Build history of the part. All positions in model axes, mm. A direction names the side the tool comes from. Round coordinates to 2 decimals unless told otherwise and drop trailing zeros. Write each loop counter-clockwise with the first axis right and the second up, starting at its lowest first coordinate (ties: lowest second). Pieces come first, ordered by that corner, then holes. Notation, with made-up numbers: (82, 73.25) - (99, 73.25) arc R36 ccw to (99, 109.25) - close; hole circle Ø3 at (-22.5, 61.5). An arc over 180 degrees is marked (long way). Answer as a JSON object with one key per item and string values. Group by question number.
Item 1: Slice it at A-A, the plane x = -105.5. List the corners of the cut face in (y, z), then the cut area to 3 significant figures.
Item 2: Flat gauge pins, fed straight in: pin 1 (2 mm diameter, centred on y = 37, z = 11.5, fed in from -X); pin 2 (1 mm diameter, centred on x = -4.5, z = 5.5, fed in from -Y); pin 3 (1.5 mm diameter, centred on x = 50.5, y = 78.5, fed in from +Z). Where does each tip first touch, or does it go through?
Item 3: Slice it at B-B, the plane z = 39. List the corners of the cut face in (x, y), then the cut area to 3 significant figures.
Item 4: Which spindle directions (+Z, -Z, +X, -X, +Y, -Y) get a long thin tool onto all of the face, cutting with end or side? Do faces 4 (the cylindrical face through (27.268, 57.226, -13.977)), 5 (the cylindrical face through (23.846, 14.79, 7.509)), 6 (the flat face through (-130, 100, 0)), 7 (the cylindrical face through (-114.79, 118.426, 16.896)). Say none if no direction does.
Item 5: Two-plate mould, pull along X, no slides. Class faces 1 (the flat face through (0, 109.6, 23.3)), 2 (the flat face through (0, 30, 0)), 3 (the flat face through (17, 0, -19)): +X half, -X half, draft (parallel to the pull), parting line (faces both ways), or undercut.
Item 6: Slice it at D-D, the plane z = 67.5. List the corners of the cut face in (x, y), then the cut area to 3 significant figures.
Item 7: Probe line 1 (Y direction, x = 23.5, z = 0); line 2 (Y direction, x = 53, z = -14); line 3 (Z direction, x = 30.5, y = 100). List the from-to ranges inside material, lowest first. Write a range as from..to.
Item 8: Slice it at C-C, the plane z = -60.5. List the corners of the cut face in (x, y).
from build123d import *

# Parameters (mm, degrees)
SWEEP2_PROFILE_R    = 80
SKETCH11_R          = 25
CUT_EXTRUDE1_DEPTH  = 30
SKETCH12_R          = 25
BOSS_EXTRUDE1_DEPTH = 30
SKETCH13_R          = 50
SKETCH13_R_2        = 45
SKETCH13_R_3        = 35
SKETCH13_R_4        = 25
CUT_EXTRUDE2_DEPTH  = 237.008474534


with BuildPart() as part:
    # Sweep2: sweep along a path in Sketch1
    with BuildLine(Plane.XY) as sweep2_path:
        ThreePointArc((0, 0), (-29.289321881, 70.710678119), (-100, 100))
    # Sweep2 profile (on start of the path) → Sweep2 (sweep)
    with BuildSketch(Plane(origin=(0, 0, 0), x_dir=(1, 0, 0), z_dir=(0, 1, 0))):
        Circle(SWEEP2_PROFILE_R)
    sweep(path=sweep2_path.line)

    # Sketch11 → Cut-Extrude1 (cut)
    with BuildSketch(Plane.XZ):
        Circle(SKETCH11_R)
    extrude(amount=-CUT_EXTRUDE1_DEPTH, mode=Mode.SUBTRACT)

    # Sketch12 → Boss-Extrude1 (add)
    with BuildSketch(Plane.ZY.offset(100)):
        with Locations(Location((0, 100, 0), (0, 0, 270))):
            Circle(SKETCH12_R)
    extrude(amount=BOSS_EXTRUDE1_DEPTH)

    # Sketch13 → Cut-Extrude2 (cut, through all)
    # profile 1 of 2: a face of its own
    with BuildSketch(Plane(origin=(0, 0, 0), x_dir=(0, 0, -1), z_dir=(1, 0, 0))):
        with Locations((0, 100)):
            Circle(SKETCH13_R)
        with Locations(Location((0, 100, 0), (0, 0, 350.615107279))):
            Circle(SKETCH13_R_2, mode=Mode.SUBTRACT)
    # profile 2 of 2: a face of its own
    with BuildSketch(Plane(origin=(0, 0, 0), x_dir=(0, 0, -1), z_dir=(1, 0, 0))):
        with Locations(Location((0, 100, 0), (0, 0, 356.680271872))):
            Circle(SKETCH13_R_3)
        with Locations(Location((0, 100, 0), (0, 0, 270))):
            Circle(SKETCH13_R_4, mode=Mode.SUBTRACT)
    extrude(amount=CUT_EXTRUDE2_DEPTH, mode=Mode.SUBTRACT)


solid = part.part
Geometry says:
{
 "1": {"outline": "circle Ø50 at (100, 0)", "area": "1,960 mm^2"},
 "2": {"pin 1": "stops at x = -100", "pin 2": "stops at y = 30", "pin 3": "stops at z = 39.77"},
 "3": {"outline": "(-100, 30.15) arc R30.15 cw to (-69.85, 0) - (69.85, 0) arc R169.85 ccw to (55.33, 68.71) - (0, 68.71) - (0, 77.55) - (51.11, 77.55) arc R169.85 ccw to (17.71, 122.45) - (0, 122.45) - (0, 131.29) - (7.76, 131.29) arc R169.85 ccw to (-100, 169.85) - close", "area": "21,400 mm^2"},
 "4": {"face 4": "+X", "face 5": "-Y", "face 6": "+Z, -Z, -X, +Y, -Y", "face 7": "-X"},
 "5": {"face 1": "+X half", "face 2": "undercut", "face 3": "draft"},
 "6": {"outline": "(-100, 57.06) arc R57.06 cw to (-42.94, 0) - (42.94, 0) arc R142.94 ccw to (-100, 142.94) - close", "area": "13,500 mm^2"},
 "7": {"line 1": "y = 30..50, 55..65, 75..125", "line 2": "y = 0..52, 57.23..67.92, 79.29..92.46", "line 3": "z = -45..-35, -25..25, 35..45"},
 "8": {"outline": "(-100, 47.66) arc R47.66 cw to (-52.34, 0) - (52.34, 0) arc R152.34 ccw to (-100, 152.34) - close"}
}
